For this review, take the finished solid that the model builds, in its own axes (mm). A direction names the side the tool comes from. Coordinates: 2 decimals unless noted, no trailing zeros. Write each loop counter-clockwise with the first axis right and the second up, starting at its lowest first coordinate (ties: lowest second). Pieces come first, ordered by that corner, then holes.
1) We need section B-B on z = 1. Write out the cut boundary in (x, y).
2) We need section A-A on x = -4. Write out the cut boundary in (y, z).
3) To check wall thickness, follow line 1 along X through (y, z) = (-3.75, 20); line 2 along Z through (x, y) = (-9.5, 5.75); line 3 along Z through (x, y) = (4, -1). State the ranges of each line that lie inside material, in increasing order.
4) We need section D-D on x = 6.25. Write out the cut boundary in (y, z), then the cut area to 3 significant figures.
5) We need section C-C on y = 8.5. Write out the cut boundary in (x, z), then the cut area to 3 significant figures.
6) For faces 1 (the face through (-3.95, -6.72, 12.33)), 2 (the face through (3.95, 6.72, 14.25)), 3 (the face through (-3.843, 6.781, 12.325)), list the 3-axis set-ups (+Z, -Z, +X, -X, +Y, -Y) from which the entire face can be reached by the end or side of a thin tool; tool diameter is ignored.
7) Insertion check: P1, Ø4, axis at x = 5.5, z = 22.5, coming from the +Y side; P2, Ø4, axis at x = -6.5, z = 9, coming from the -Y side; P3, Ø7, axis at y = -1.5, z = 9.5, coming from the +X side; P4, Ø12, axis at x = 3.5, y = 2, coming from the +Z side. Each pin has a flat end and moves straight along its axis. Give the tip position at first contact, or say it passes through.
from build123d import *

# Parameters (mm, degrees)
SALIENTE_EXTRUIR1_DEPTH = 30
CROQUIS2_R              = 12
SALIENTE_EXTRUIR2_DEPTH = 2
CHAMFER1_SIZE           = 5


with BuildPart() as part:
    # Croquis1 → Saliente-Extruir1 (new body)
    with BuildSketch(Plane.XY):
        Polygon((0, 9), (-7.794228634, 4.5), (-7.794228634, -4.5), (0, -9), (7.794228634, -4.5), (7.794228634, 4.5), align=None)
    extrude(amount=SALIENTE_EXTRUIR1_DEPTH)

    # Croquis2 → Saliente-Extruir2 (add)
    with BuildSketch(Plane(origin=(0, 0, 0), x_dir=(-1, 0, 0), z_dir=(0, 0, -1))):
        Circle(CROQUIS2_R)
    extrude(amount=SALIENTE_EXTRUIR2_DEPTH)

    # Chamfer1
    # the kernel refuses this chamfer: 5 mm, written as the material it takes off along each edge
    with BuildSketch(Plane(origin=(-18.929942624, 1.92920747, 30), x_dir=(-0.013747938305293065, -0.023812127644090277, -0.9996219169112968), z_dir=(0.8660254037844416, -0.49999999999999495, 0)), Plane(origin=(7.794228634, -17.35841494, 30), x_dir=(0.027495876610586317, 0, -0.9996219169112968), z_dir=(0, 1, 0)), Plane(origin=(11.13571399, 15.42920747, 30), x_dir=(-0.013747938305293275, 0.023812127644090242, -0.9996219169112968), z_dir=(-0.8660254037844379, -0.5000000000000012, 0))) as chamfer1_piece_1:
        Polygon((CHAMFER1_SIZE * 0.999621916911, CHAMFER1_SIZE * 0.0274958766106), (-CHAMFER1_SIZE * 0.0274958766106, CHAMFER1_SIZE * 0.999621916911), (0, 0), align=None)
    extrude(amount=34.71682988, mode=Mode.SUBTRACT)


solid = part.part
Result:
1. outline: (-7.79, -4.5) - (0, -9) - (7.79, -4.5) - (7.79, 4.5) - (0, 9) - (-7.79, 4.5) - close
2. outline: (-11.31, -2) - (11.31, -2) - (11.31, 0) - (6.69, 0) - (6.69, 25) - (0.92, 30) - (-0.92, 30) - (-6.69, 25) - (-6.69, 0) - (-11.31, 0) - close
3. line 1: x = -7.79 to 7.79
3. line 2: z = -2 to 0
3. line 3: z = -2 to 28.79
4. outline: (-10.24, -2) - (10.24, -2) - (10.24, 0) - (5.39, 0) - (5.39, 26.54) - (-5.39, 26.54) - (-5.39, 0) - (-10.24, 0) - close
4. area: 327 mm2
5. outline: (-8.47, -2) - (8.47, -2) - (8.47, 0) - (0.87, 0) - (0.87, 25.87) - (-0.87, 25) - (-0.87, 0) - (-8.47, 0) - close
5. area: 77.9 mm2
6. face 1: +Z, -X, -Y
6. face 2: +Z, +X, +Y
6. face 3: +Z, -X, +Y
7. P1: stops at y = 6.98
7. P2: stops at y = -6.4
7. P3: stops at x = 7.79
7. P4: stops at z = 30
